Autodesk Inventor part; units mm, degrees
ref_plane "YZ Plane" through (0, 0, 0) normal (1, 0, 0) x (0, 1, 0)
ref_plane "XZ Plane" through (0, 0, 0) normal (0, 1, 0) x (-1, 0, 0)
ref_plane "XY Plane" through (0, 0, 0) normal (0, 0, 1) x (1, 0, 0)
sketch "Sketch1" plane through (0, 0, 0) normal (0, 1, 0) x (-1, 0, 0)
  line L0 (63, 23.25) -> (-67, 23.25)
  line L1 (-67, 23.25) -> (-67, -23.25)
  line L2 (-67, -23.25) -> (63, -23.25)
  line L3 (63, -23.25) -> (63, 23.25)
  point P0 (0, 0)
  dimension "d1" = 46.5
  dimension "d2" = 23.25
  dimension "d3" = 130
  dimension "d4" = 67
extrude "Extrusion1" add sketch "Sketch1" along normal blind 3.5
sketch "Sketch3" plane through (0, 3.5, 0) normal (0, 1, 0) x (1, 0, 0)
  line L0 (-58, 6.75) -> (-47, 6.75)
  line L1 (-47, 6.75) -> (-47, -6.75)
  line L2 (-47, -6.75) -> (-58, -6.75)
  line L3 (-58, -6.75) -> (-58, 6.75)
  line L4 (-37, 6.75) -> (-25, 6.75)
  line L5 (-25, 6.75) -> (-25, -6.75)
  line L6 (-25, -6.75) -> (-37, -6.75)
  line L7 (-37, -6.75) -> (-37, 6.75)
  line L8 (-15, 6.75) -> (-3, 6.75)
  line L9 (-3, 6.75) -> (-3, -6.75)
  line L10 (-3, -6.75) -> (-15, -6.75)
  line L11 (-15, -6.75) -> (-15, 6.75)
  line L12 (7, 6.75) -> (19, 6.75)
  line L13 (19, 6.75) -> (19, -6.75)
  line L14 (19, -6.75) -> (7, -6.75)
  line L15 (7, -6.75) -> (7, 6.75)
  line L16 (29, 6.75) -> (41, 6.75)
  line L17 (41, 6.75) -> (41, -6.75)
  line L18 (41, -6.75) -> (29, -6.75)
  line L19 (29, -6.75) -> (29, 6.75)
  line L20 (51, 6.75) -> (62, 6.75)
  line L21 (62, 6.75) -> (62, -6.75)
  line L22 (62, -6.75) -> (51, -6.75)
  line L23 (51, -6.75) -> (51, 6.75)
  line L24 (67, 23.25) -> (-63, 23.25)
  line L25 (-63, -23.25) -> (67, -23.25)
  line L26 (-63, 23.25) -> (-63, -23.25)
  line L27 (67, -23.25) -> (67, 23.25)
  point P0 (0, 0)
  dimension "d21" = 16.5
  dimension "d22" = 16.5
  dimension "d23" = 5
  dimension "d24" = 10
  dimension "d25" = 10
  dimension "d26" = 10
  dimension "d27" = 10
  dimension "d28" = 5
  dimension "d29" = 16
  dimension "d30" = 38
  dimension "d31" = 60
  dimension "d32" = 60
  dimension "d33" = 38
  dimension "d34" = 16
extrude "Extrusion3" cut sketch "Sketch3" against normal blind 10 contours L0 L1 L2 L3 | L4 L5 L6 L7 | L8 L9 L10 L11 | L12 L13 L14 L15 | L16 L17 L18 L19 | L20 L21 L22 L23
sketch "Sketch4" plane through (0, 3.5, 0) normal (0, 1, 0) x (1, 0, 0)
  point P0 (0, 0)
sketch "Sketch5" plane through (0, 3.5, 0) normal (0, 1, 0) x (1, 0, 0)
  circle A0 centre (0, 16.25) radius 2.25
  circle A1 centre (0, -16.25) radius 2.25
  line L0 (67, 23.25) -> (-63, 23.25)
  line L1 (67, -23.25) -> (67, 23.25)
  line L2 (-63, -23.25) -> (67, -23.25)
  point P0 (0, 0)
  dimension "d37" = 4.5
  dimension "d38" = 4.5
  dimension "d39" = 7
  dimension "d40" = 67
  dimension "d41" = 7
  dimension "d42" = 67
extrude "Extrusion4" cut sketch "Sketch5" against normal blind 3.5
properties part number "MILESTONE3LID"
Geometry: final body of the model. Coordinates: model frame, mm. A direction names the side the tool comes from. Round coordinates to 2 decimals unless told otherwise and drop trailing zeros. Order: outer loops, then holes, each group sorted by start corner. A loop starts at its lowest first (then second) coordinate and runs counter-clockwise, first axis right, second up. Notation, with made-up numbers: (-22, 63.5) -> (12, 63.5) arc R18 ccw to (12, 72.5) -> close; hole circle Ø2 at (18.25, -23.5). An arc over 180 degrees is marked (long way). Use one line per item in the form item = value. Start each with the question number.
1. Cut plane C-C (z = -2.5). Return the cut outline in (x, y).
2. Cut plane B-B (x = 39). Return the cut outline in (y, z).
3. Draft query along Z for faces 3 (the face through (1, 2, 23.25)), 4 (the face through (-9, 2, 6.75)), 5 (the face through (3, 3.5, 0)), 6 (the face through (-31, 2, -6.75)). Return one class per face: pulls with the +Z half, pulls with the -Z half, needs draft (parallel to the pull), parting line crosses it, or undercut.
4. Line query: probe 1 along Z at (x, y) = (0, 2.2); probe 2 along Z at (x, y) = (37.5, 1.35); probe 3 along X at (y, z) = (2.5, -16.25). Output: solid intervals per line, ascending.
5. Cut plane D-D (y = 2.55). Count the separate pieces of the cut face and the enclosed holes in it, then the cut area to 3 significant figures.
6. Reachability of faces 1 (the face through (-63, 2, 0)), 2 (the face through (35, 2, -6.75)) from +Z, -Z, +X, -X, +Y, -Y: full face, straight path, thin tool, end or side. Return the list, or none.
7. Cut plane A-A (z = 16.25). Return the cut outline in (x, y), then the cut area to 3 significant figures.
Solution:
q1.outline = (-63, 0) -> (-58, 0) -> (-58, 3.5) -> (-63, 3.5) -> close; (-47, 0) -> (-37, 0) -> (-37, 3.5) -> (-47, 3.5) -> close; (-25, 0) -> (-15, 0) -> (-15, 3.5) -> (-25, 3.5) -> close; (-3, 0) -> (7, 0) -> (7, 3.5) -> (-3, 3.5) -> close; (19, 0) -> (29, 0) -> (29, 3.5) -> (19, 3.5) -> close; (41, 0) -> (51, 0) -> (51, 3.5) -> (41, 3.5) -> close; (62, 0) -> (67, 0) -> (67, 3.5) -> (62, 3.5) -> close
q2.outline = (0, -23.25) -> (3.5, -23.25) -> (3.5, -6.75) -> (0, -6.75) -> close; (0, 6.75) -> (3.5, 6.75) -> (3.5, 23.25) -> (0, 23.25) -> close
q3.face_3 = pulls with the +Z half
q3.face_4 = undercut
q3.face_5 = needs draft
q3.face_6 = undercut
q4.probe_1 = -23.25 to -18.5, -14 to 14, 18.5 to 23.25
q4.probe_2 = -23.25 to -6.75, 6.75 to 23.25
q4.probe_3 = -63 to -2.25, 2.25 to 67
q5.separate_pieces = 1
q5.enclosed_holes = 8
q5.area = 5,070 mm^2
q6.face_1 = +Z, -Z, -X, +Y, -Y
q6.face_2 = +Y, -Y
q7.outline = (-63, 0) -> (-2.25, 0) -> (-2.25, 3.5) -> (-63, 3.5) -> close; (2.25, 0) -> (67, 0) -> (67, 3.5) -> (2.25, 3.5) -> close
q7.area = 439 mm^2
